The listing builds one solid part. Answer for the finished solid, in the listing's coordinates (mm). A direction names the side the tool comes from. Give positions to 0.01 mm unless a question says otherwise; leave off trailing zeros. Loops run counter-clockwise (first coordinate to the right, second up) from the corner with the lowest first, then second, coordinate; pieces in that order, holes last. Notation, with made-up numbers: M -5,38.25 L 46,38.25 A27 cw 46,63.25 Z; hole C -17.75,54.5 d2. An arc over 180 degrees is marked long. Return JSON: item names as keys, results as strings.
from build123d import *

# Parameters (mm, degrees)
F0_R     = 2.75
F0_W     = 1.85
F0_H     = 10.75
F0_W_2   = 10
F1_DEPTH = 12.7


# Not quite as in the source:
# - a length typed as a fraction of an inch, garbled in the dataset ("3 / 203.2 mm" for 3/8 in), is restored


with BuildPart() as f1:
    # F0 (on Top) → F1 (new body)
    with BuildSketch(Plane.XY):
        Polygon((-15.75, -14.25), (-15.75, -25), (-6.85, -25), (-6.85, -14.25), (-9.85, -14.25), align=None)
        with Locations((-10, -20)):
            Circle(F0_R, mode=Mode.SUBTRACT)
        with Locations((-5.925, -19.625)):
            Rectangle(F0_W, F0_H)
        with Locations((0, -19.625)):
            Rectangle(F0_W_2, F0_H)
        with BuildLine():
            Line((-9.85, -14.25), (-6.85, -14.25))
            Line((-6.85, -14.25), (-6.85, 0))
            ThreePointArc((-6.85, 0), (0, 6.85), (6.85, 0))
            Line((6.85, 0), (6.85, -14.25))
            Line((6.85, -14.25), (9.85, -14.25))
            Line((9.85, -14.25), (9.85, 9.85))
            Line((9.85, 9.85), (-9.85, 9.85))
            Line((-9.85, 9.85), (-9.85, -14.25))
        make_face()
        with Locations((5.925, -19.625)):
            Rectangle(F0_W, F0_H)
        Polygon((6.85, -14.25), (6.85, -25), (15.75, -25), (15.75, -14.25), (9.85, -14.25), align=None)
        with Locations((10, -20)):
            Circle(F0_R, mode=Mode.SUBTRACT)
        with BuildLine():
            Line((-6.85, 0), (-6.85, -14.25))
            Line((-6.85, -14.25), (-5, -14.25))
            Line((-5, -14.25), (-5, -4.6821469434))
            ThreePointArc((-5, -4.6821469434), (-6.3707338667, -2.5171908946), (-6.85, 0))
        make_face()
        with BuildLine():
            Line((5, -4.6821469434), (5, -14.25))
            Line((5, -14.25), (6.85, -14.25))
            Line((6.85, -14.25), (6.85, 0))
            ThreePointArc((6.85, 0), (6.3707338667, -2.5171908946), (5, -4.6821469434))
        make_face()
        with BuildLine():
            Line((-5, -4.6821469434), (-5, -14.25))
            Line((-5, -14.25), (5, -14.25))
            Line((5, -14.25), (5, -4.6821469434))
            ThreePointArc((5, -4.6821469434), (0, -6.85), (-5, -4.6821469434))
        make_face()
    extrude(amount=-F1_DEPTH)


solid = f1.part
(1) The part is cut by section D-D (y = -2.5). Determine the outline of the cut face in (x, z), and give its area (3 significant figures).
Values follow:
{"outline": "M -9.85,-12.7 L -6.38,-12.7 L -6.38,0 L -9.85,0 Z; M 6.38,-12.7 L 9.85,-12.7 L 9.85,0 L 6.38,0 Z", "area": "88.2 mm²"}
(2) Given pin 1 (6.5 mm diameter, centred on x = 14, z = -3.5, fed in from +Y); pin 2 (6.5 mm diameter, centred on y = -3, z = -6, fed in from +X), each flat-ended and moving along its own axis, determine where each tip first touches the part or whether it passes through.
Values follow:
{"pin 1": "y = -14.25", "pin 2": "x = 9.85"}
(3) The part is cut by section C-C (x = 0). Determine the outline of the cut face in (y, z), and give its area (3 significant figures).
Values follow:
{"outline": "M -25,-12.7 L -6.85,-12.7 L -6.85,0 L -25,0 Z; M 6.85,-12.7 L 9.85,-12.7 L 9.85,0 L 6.85,0 Z", "area": "269 mm²"}
(4) Straight lines are drawn through the part: line 1 along Y through (x, z) = (10, -5.5); line 2 along X through (y, z) = (-21.5, -1.5); line 3 along X through (y, z) = (-13.5, -9). For each, find the intervals that lie inside material, in ascending order.
Values follow:
{"line 1": "-25 to -22.75, -17.25 to -14.25", "line 2": "-15.75 to -12.3, -7.7 to 7.7, 12.3 to 15.75", "line 3": "-9.85 to 9.85"}
(5) Determine the mould class of faces 1 (the cylindrical face through (9.642, -17.273, -6.261)), 2 (the flat face through (-13, -14.25, -6)), 3 (the flat face through (15.75, -20, -6)), 4 (the cylindrical face through (-10.358, -17.273, -6.261)) for opening direction X: released by +X, released by -X, zero draft, split by the parting line, or undercut.
Values follow:
{"face 1": "undercut", "face 2": "zero draft", "face 3": "released by +X", "face 4": "undercut"}
(6) A tool of negligible diameter and unlimited length cuts with its end or side. For faces 5 (the flat face through (-15.75, -20, -6)), 6 (the flat face through (13, -14.25, -6)), 7 (the flat face through (-9.85, -2, -6)), from which of +Z, -Z, +X, -X, +Y, -Y can it reach the whole face along a straight path? Write none if from no direction.
Values follow:
{"face 5": "+Z, -Z, -X, +Y, -Y", "face 6": "+Z, -Z, +X, +Y", "face 7": "+Z, -Z, -X, +Y"}
(7) The part is cut by section A-A (y = -20). Determine the outline of the cut face in (x, z), and give its area (3 significant figures).
Values follow:
{"outline": "M -15.75,-12.7 L -12.75,-12.7 L -12.75,0 L -15.75,0 Z; M -7.25,-12.7 L 7.25,-12.7 L 7.25,0 L -7.25,0 Z; M 12.75,-12.7 L 15.75,-12.7 L 15.75,0 L 12.75,0 Z", "area": "260 mm²"}
(8) The part is cut by section B-B (z = -5.75). Determine the outline of the cut face in (x, y).
Values follow:
{"outline": "M -15.75,-25 L 15.75,-25 L 15.75,-14.25 L 9.85,-14.25 L 9.85,9.85 L -9.85,9.85 L -9.85,-14.25 L -15.75,-14.25 Z; hole C -10,-20 d5.5; hole C 0,0 d13.7; hole C 10,-20 d5.5"}
